CAD build for the part. Positions are in the model's coordinates, mm. A direction names the side the tool comes from. Coordinates: 2 decimals unless noted, no trailing zeros. Write each loop counter-clockwise with the first axis right and the second up, starting at its lowest first coordinate (ties: lowest second). Pieces come first, ordered by that corner, then holes. Notation, with made-up numbers: (29.25, 57.5) - (56.25, 57.5) arc R17 cw to (56.25, 70.5) - close; hole circle Ø2 at (71, -11). An arc over 180 degrees is marked (long way). Answer in a Markdown table with one row per item. Add a question column.
Q1. 3-axis set-ups, long thin cutter, end or side, ignore diameter. For faces 4 (the cylindrical face through (0.032, 6.466, 2.681)), 5 (the cylindrical face through (-1.951, 6.466, 2.681)), 6 (the cylindrical face through (-3.918, 6.466, 2.681)): which of +Z, -Z, +X, -X, +Y, -Y reach the whole face in a straight line?
Q2. Two-plate mould, pull along X, no slides. Class faces 1 (the cylindrical face through (-0.69, -5.75, -5.27)), 2 (the flat face through (-4.437, -2, -6)), 3 (the flat face through (-2.937, 6, -4)): +X half, -X half, draft (parallel to the pull), parting line (faces both ways), or undercut.
Q3. Pin check, flat tips, straight feed: pin 1 (8 mm diameter, centred on y = -1.5, z = -3, fed in from -X); pin 2 (1 mm diameter, centred on x = -2.5, z = -2.5, fed in from -Y). Stop position of each tip, or through.
Q4. Band-saw the part on C-C (x = -2). List the corners of the cut face in (y, z), and give its area (3 significant figures).
Q5. Drill centre lines: line 1 along Y through (x, z) = (-0.55, 0); line 2 along Y through (x, z) = (-1.4, 0). Where is each one in solid material? Low to high. Write a range as from..to.
```python
from build123d import *

# Parameters (mm, degrees)
SMUSSO1_SIZE = 0.05


with BuildPart() as part:
    # Schizzo1 → Rivoluzione1 (revolve)
    with BuildSketch(Plane.XY):
        Polygon((-4.436619718, 6), (0.563380282, 6), (0.563380282, 7), (-0.436619718, 7), (-0.436619718, 7.8), (-0.936619718, 7.8), (-0.936619718, 7), (-2.936619718, 7), (-2.936619718, 7.8), (-3.436619718, 7.8), (-3.436619718, 7), (-4.436619718, 7), align=None)
    revolve(axis=Axis((0, 0, 0), (-1, 0, 0)))

    # Smusso1
    smusso1_edges = [part.edges().sort_by_distance(p)[0] for p in [
        (0.563380282, -7, 0),
        (0.563380282, -6, 0),
        (-4.436619718, -6, 0),
        (-4.436619718, -7, 0),
    ]]
    chamfer(smusso1_edges, length=SMUSSO1_SIZE)


solid = part.part
```
Checked values:
| question | item | result |
|---|---|---|
| 1 | face 4 | +X |
| 1 | face 5 | none |
| 1 | face 6 | -X |
| 2 | face 1 | draft |
| 2 | face 2 | -X half |
| 2 | face 3 | undercut |
| 3 | pin 1 | stops at x = -4.44 |
| 3 | pin 2 | stops at y = -7.47 |
| 4 | outline | circle Ø14 at (0, 0); hole circle Ø12 at (0, 0) |
| 4 | area | 40.8 mm² |
| 5 | line 1 | y = -7.8..-6, 6..7.8 |
| 5 | line 2 | y = -7..-6, 6..7 |
